from build123d import *

# Parameters (mm, degrees)
BOSS_EXTRUDE1_DEPTH        = 75
M6X1_0_TAPPED_HOLE1_REACH  = 111.972
M6X1_0_TAPPED_HOLE1_BORE_R = 2.5
M6X1_0_TAPPED_HOLE2_D      = 5
SKETCH8_R                  = 2.6
CUT_EXTRUDE1_DEPTH         = 110.972346069
SKETCH9_W                  = 10
SKETCH9_H                  = 31.74
BOSS_EXTRUDE2_DEPTH        = 32
CUT_EXTRUDE2_REACH         = 128.008
SKETCH10_R                 = 2.1
BOSS_EXTRUDE3_DEPTH        = 10
M6X1_0_TAPPED_HOLE3_D      = 5
M6X1_0_TAPPED_HOLE3_DEPTH  = 13.851
FILLET1_R                  = 3.175
CHAMFER1_SIZE              = 5
FILLET2_R                  = 2.5
FILLET3_R                  = 1.5


with BuildPart() as part:
    # Sketch1 → Boss-Extrude1 (new body)
    with BuildSketch(Plane.XY):
        Polygon((6.35, 33.52), (13.85, 41.02), (51.15, 41.02), (58.65, 33.52), (58.65, 0), (65, 0), (65, 41.02), (65, 47.37), (0, 47.37), (0, 41.02), (0, 0), (6.35, 0), align=None)
    extrude(amount=BOSS_EXTRUDE1_DEPTH)

    # M6x1.0 Tapped Hole1 bore → M6x1.0 Tapped Hole1 (cut, up to next)
    with BuildSketch(Plane.ZY, mode=Mode.PRIVATE) as m6x1_0_tapped_hole1_sk1:
        with Locations((60, 15.87)):
            Circle(M6X1_0_TAPPED_HOLE1_BORE_R)
    m6x1_0_tapped_hole1_tool1 = extrude(m6x1_0_tapped_hole1_sk1.sketch, amount=-M6X1_0_TAPPED_HOLE1_REACH, mode=Mode.PRIVATE) & part.part
    # M6x1.0 Tapped Hole1 bore → M6x1.0 Tapped Hole1 (cut, up to next)
    with BuildSketch(Plane.ZY, mode=Mode.PRIVATE) as m6x1_0_tapped_hole1_sk2:
        with Locations((15, 15.87)):
            Circle(M6X1_0_TAPPED_HOLE1_BORE_R)
    m6x1_0_tapped_hole1_tool2 = extrude(m6x1_0_tapped_hole1_sk2.sketch, amount=-M6X1_0_TAPPED_HOLE1_REACH, mode=Mode.PRIVATE) & part.part
    m6x1_0_tapped_hole1_1 = m6x1_0_tapped_hole1_tool1.solids().sort_by_distance((0, 15.87, 60))[0]
    add(m6x1_0_tapped_hole1_1, mode=Mode.SUBTRACT)
    m6x1_0_tapped_hole1_2 = m6x1_0_tapped_hole1_tool2.solids().sort_by_distance((0, 15.87, 15))[0]
    add(m6x1_0_tapped_hole1_2, mode=Mode.SUBTRACT)
    m6x1_0_tapped_hole1 = m6x1_0_tapped_hole1_1 + m6x1_0_tapped_hole1_2  # M6x1.0 Tapped Hole1 as one shape, for the pattern or mirror that repeats it

    # Mirror1: M6x1.0 Tapped Hole1 across plane
    add(m6x1_0_tapped_hole1.mirror(Plane.ZY.offset(-32.5)), mode=Mode.SUBTRACT)

    # M6x1.0 Tapped Hole2 (through all)
    with Locations(Plane(origin=(0, 47.37, 0), x_dir=(1, 0, 0), z_dir=(0, 1, 0))):
        with Locations((32.5, -15), (32.5, -60)):
            Hole(M6X1_0_TAPPED_HOLE2_D / 2)

    # Sketch8 → Cut-Extrude1 (cut, through all)
    with BuildSketch(Plane.ZY):
        with Locations((37.5, 15.87)):
            Circle(SKETCH8_R)
    extrude(amount=-CUT_EXTRUDE1_DEPTH, mode=Mode.SUBTRACT)

    # Sketch9 → Boss-Extrude2 (add)
    with BuildSketch(Plane(origin=(65, 0, 0), x_dir=(0, 0, -1), z_dir=(1, 0, 0))):
        with Locations((-70, 15.87)):
            Rectangle(SKETCH9_W, SKETCH9_H)
    extrude(amount=BOSS_EXTRUDE2_DEPTH)

    # Sketch10 → Cut-Extrude2 (cut, up to next)
    with BuildSketch(Plane(origin=(0, 0, 65), x_dir=(-1, 0, 0), z_dir=(0, 0, -1)), mode=Mode.PRIVATE) as cut_extrude2_sk1:
        with Locations((-87, 28.87)):
            Circle(SKETCH10_R)
    cut_extrude2_tool1 = extrude(cut_extrude2_sk1.sketch, amount=-CUT_EXTRUDE2_REACH, mode=Mode.PRIVATE) & part.part
    # Sketch10 → Cut-Extrude2 (cut, up to next)
    with BuildSketch(Plane(origin=(0, 0, 65), x_dir=(-1, 0, 0), z_dir=(0, 0, -1)), mode=Mode.PRIVATE) as cut_extrude2_sk2:
        with Locations((-87, 2.87)):
            Circle(SKETCH10_R)
    cut_extrude2_tool2 = extrude(cut_extrude2_sk2.sketch, amount=-CUT_EXTRUDE2_REACH, mode=Mode.PRIVATE) & part.part
    # Sketch10 → Cut-Extrude2 (cut, up to next)
    with BuildSketch(Plane(origin=(0, 0, 65), x_dir=(-1, 0, 0), z_dir=(0, 0, -1)), mode=Mode.PRIVATE) as cut_extrude2_sk3:
        with BuildLine():
            Line((-87, 26.07), (-97, 26.07))
            Line((-97, 26.07), (-97, 5.67))
            Line((-97, 5.67), (-87, 5.67))
            ThreePointArc((-87, 5.67), (-76.8, 15.87), (-87, 26.07))
        make_face()
    cut_extrude2_tool3 = extrude(cut_extrude2_sk3.sketch, amount=-CUT_EXTRUDE2_REACH, mode=Mode.PRIVATE) & part.part
    add(cut_extrude2_tool1.solids().sort_by_distance((87, 28.87, 65))[0], mode=Mode.SUBTRACT)
    add(cut_extrude2_tool2.solids().sort_by_distance((87, 2.87, 65))[0], mode=Mode.SUBTRACT)
    add(cut_extrude2_tool3.solids().sort_by_distance((87.850588, 15.87, 65))[0], mode=Mode.SUBTRACT)

    # Sketch11 → Boss-Extrude3 (add)
    with BuildSketch(Plane.XY.offset(75)):
        Polygon((97, 31.74), (65, 42.87), (65, 31.74), align=None)
    extrude(amount=-BOSS_EXTRUDE3_DEPTH)

    # M6x1.0 Tapped Hole3
    with Locations(Plane(origin=(0, 47.37, 0), x_dir=(1, 0, 0), z_dir=(0, 1, 0))):
        with Locations((54.9, -57.5), (54.9, -37.5), (54.9, -17.5)):
            m6x1_0_tapped_hole3 = Hole(M6X1_0_TAPPED_HOLE3_D / 2, depth=M6X1_0_TAPPED_HOLE3_DEPTH)

    # Mirror2: M6x1.0 Tapped Hole3 across plane
    add(m6x1_0_tapped_hole3.mirror(Plane.ZY.offset(-32.5)), mode=Mode.SUBTRACT)

    # Fillet1
    # the kernel refuses this fillet: 3.175 mm, written as the material it takes off along each edge
    with BuildSketch(Plane(origin=(97, 5.67, 57.0625), x_dir=(0, -1, 0), z_dir=(0, 0, 1)), Plane(origin=(97, 26.07, 57.0625), x_dir=(-1, 0, 0), z_dir=(0, 0, 1))) as fillet1_piece_1:
        with BuildLine():
            CenterArc((FILLET1_R, -FILLET1_R), FILLET1_R, 90, 90)
            Line((0, -FILLET1_R), (0, 0))
            Line((0, 0), (FILLET1_R, 0))
        make_face()
    extrude(amount=25.875, mode=Mode.SUBTRACT)
    with BuildSketch(Plane(origin=(97, 31.74, 59.356851229), x_dir=(0, -1, 0), z_dir=(0, 0, 1))) as fillet1_piece_2:
        with BuildLine():
            CenterArc((FILLET1_R * 0.710947876646, -FILLET1_R), FILLET1_R, 90, 70.821686435)
            Line((-FILLET1_R * 0.233552901866, -FILLET1_R * 0.671490822974), (0, 0))
            Line((0, 0), (FILLET1_R * 0.710947876646, 0))
        make_face()
    extrude(amount=21.286297542, mode=Mode.SUBTRACT)
    with BuildSketch(Plane(origin=(97, 0, 82.9375), x_dir=(-1, 0, 0), z_dir=(0, 0, -1))) as fillet1_piece_3:
        with BuildLine():
            CenterArc((FILLET1_R, FILLET1_R), FILLET1_R, 180, 90)
            Line((0, FILLET1_R), (0, 0))
            Line((0, 0), (FILLET1_R, 0))
        make_face()
    extrude(amount=25.875, mode=Mode.SUBTRACT)

    # Chamfer1
    chamfer1_edges = [part.edges().sort_by_distance(p)[0] for p in [
        (0, 47.37, 37.5),
        (65, 47.37, 37.5),
    ]]
    chamfer(chamfer1_edges, length=CHAMFER1_SIZE)

    # Fillet2
    fillet2_edges = [part.edges().sort_by_distance(p)[0] for p in [
        (0, 42.37, 37.5),
        (60, 47.37, 37.5),
        (5, 47.37, 37.5),
        (65, 42.37, 32.5),
        (58.65, 33.52, 37.5),
        (51.15, 41.02, 37.5),
        (13.85, 41.02, 37.5),
        (6.35, 33.52, 37.5),
    ]]
    fillet(fillet2_edges, radius=FILLET2_R)

    # Fillet3
    fillet3_edges = [part.edges().sort_by_distance(p)[0] for p in [
        (0, 0, 37.5),
        (58.65, 0, 37.5),
        (6.35, 0, 37.5),
        (65, 0, 32.5),
    ]]
    fillet(fillet3_edges, radius=FILLET3_R)


solid = part.part
Check sheet for the modelled part. Datum: model origin and axes. Units: mm. A direction names the side the tool comes from. Coordinates: 2 decimals unless noted, no trailing zeros. Write each loop counter-clockwise with the first axis right and the second up, starting at its lowest first coordinate (ties: lowest second). Pieces come first, ordered by that corner, then holes. Notation, with made-up numbers: M 53.25,-6 L 101.25,-6 A33 ccw 101.25,33 Z; hole C 87,-18.5 d6. An arc over 180 degrees is marked long. Answer as CSV lines item,"result".
Q1. Cross-section at C-C (y = 10.5). Record the boundary of the cut face in (x, z).
Check result:
outline,"M 0,0 L 6.35,0 L 6.35,75 L 0,75 Z; M 58.65,0 L 65,0 L 65,65 L 78.33,65 L 78.33,75 L 58.65,75 Z"
Q2. Cross-section at A-A (x = 32.5). Record the boundary of the cut face in (y, z), then the cut area to 3 significant figures.
Check result:
outline,"M 41.02,0 L 47.37,0 L 47.37,12.5 L 41.02,12.5 Z; M 41.02,17.5 L 47.37,17.5 L 47.37,57.5 L 41.02,57.5 Z; M 41.02,62.5 L 47.37,62.5 L 47.37,75 L 41.02,75 Z"
area,"413 mm^2"
Q3. Mould release check, pull along X, two halves, no side actions. Record for faces 4 (the face through (3, 0, 37)), 5 (the face through (89.1, 28.96, 69.93)), 6 (the face through (95.971, 4.835, 69.93)): released by +X, released by -X, zero draft, split by the parting line, or undercut.
Check result:
face 4,"zero draft"
face 5,"undercut"
face 6,"released by +X"
Q4. Set-up check for faces 1 (the face through (90, 26.07, 70)), 2 (the face through (65, 21, 32)), 3 (the face through (58.65, 21, 37)): record each of +Z, -Z, +X, -X, +Y, -Y from which the full face is reachable in a straight line by a thin tool's end or side.
Check result:
face 1,"+Z, -Z, +X"
face 2,"-Z, +X, +Y, -Y"
face 3,"+Z, -Z, -Y"
Q5. Cross-section at D-D (x = 10.1). Record the boundary of the cut face in (y, z).
Check result:
outline,"M 37.27,0 L 47.37,0 L 47.37,15 L 37.27,15 Z; M 37.27,20 L 47.37,20 L 47.37,35 L 37.27,35 Z; M 37.27,40 L 47.37,40 L 47.37,55 L 37.27,55 Z; M 37.27,60 L 47.37,60 L 47.37,75 L 37.27,75 Z"
Q6. Cross-section at B-B (y = 15.87). Count the separate pieces of the cut face and the enclosed holes in it, then the cut area to 3 significant figures.
Check result:
separate pieces,"8"
enclosed holes,"0"
area,"877 mm^2"
Q7. Go/stop test with flat-tipped pins: pin 1 (4 mm diameter, centred on y = 15.87, z = 60, fed in from -X); pin 2 (4 mm diameter, centred on y = 32.5, z = 37.5, fed in from +X); pin 3 (6 mm diameter, centred on x = 54.9, z = 17.5, fed in from +Y); pin 4 (3 mm diameter, centred on x = 74, y = 16.5, fed in from -Z). Record where each tip stops, or that it passes through.
Check result:
pin 1,"through"
pin 2,"x = 65"
pin 3,"y = 47.37"
pin 4,"z = 65"
Q8. Material ranges on probe 1 along X at (y, z) = (17, 45.5); probe 2 along X at (y, z) = (44, 57); probe 3 along X at (y, z) = (28, 67), recorded low to high. Write a range as from..to.
Check result:
probe 1,"0..6.35, 58.65..65"
probe 2,"1.63..7.65, 12.55..52.45, 57.35..63.37"
probe 3,"0..6.35, 58.65..85.09, 88.91..96.75"
